The model under review builds one solid part; all positions refer to its coordinate system, in mm. A direction names the side the tool comes from. Round coordinates to 2 decimals unless told otherwise and drop trailing zeros. Write each loop counter-clockwise with the first axis right and the second up, starting at its lowest first coordinate (ties: lowest second). Pieces come first, ordered by that corner, then holes. Notation, with made-up numbers: (66, -40) - (70, -40) arc R30 cw to (70, -7) - close; hole circle Ø7 at (-5, -20.75). An arc over 180 degrees is marked (long way). One line per question, with ' | ' between items. Start each with the question number.
```python
from build123d import *

# Parameters (mm, degrees)
TABAN_FLAN_1_DEPTH = 10


# Sheet-metal steps are written as plain solids
with BuildPart() as part:
    # Çizim1 → Taban-Flanş1 (new body)
    with BuildSketch(Plane.XY):
        with BuildLine():
            Line((400, -35), (-400, -35))
            Line((-400, -35), (-400, 5))
            ThreePointArc((-400, 5), (-391.213203436, 26.213203436), (-370, 35))
            Line((-370, 35), (370, 35))
            ThreePointArc((370, 35), (391.213203436, 26.213203436), (400, 5))
            Line((400, 5), (400, -35))
        make_face()
        with BuildLine():
            Line((351, 20), (89, 20))
            ThreePointArc((89, 20), (75.564971157, 14.435028843), (70, 1))
            Line((70, 1), (70, -1))
            ThreePointArc((70, -1), (75.564971157, -14.435028843), (89, -20))
            Line((89, -20), (351, -20))
            ThreePointArc((351, -20), (364.435028843, -14.435028843), (370, -1))
            Line((370, -1), (370, 1))
            ThreePointArc((370, 1), (364.435028843, 14.435028843), (351, 20))
        make_face(mode=Mode.SUBTRACT)
        with BuildLine():
            Line((-70, 1), (-70, -1))
            ThreePointArc((-70, -1), (-75.564971157, -14.435028843), (-89, -20))
            Line((-89, -20), (-351, -20))
            ThreePointArc((-351, -20), (-364.435028843, -14.435028843), (-370, -1))
            Line((-370, -1), (-370, 1))
            ThreePointArc((-370, 1), (-364.435028843, 14.435028843), (-351, 20))
            Line((-351, 20), (-89, 20))
            ThreePointArc((-89, 20), (-75.564971157, 14.435028843), (-70, 1))
        make_face(mode=Mode.SUBTRACT)
    extrude(amount=-TABAN_FLAN_1_DEPTH)


solid = part.part
```
1. Add section B-B, the plane z = -2.75. Write out the cut boundary in (x, y).
2. Wall thickness on line 1 along X through (y, z) = (-0.5, -3.5); line 2 along Y through (x, z) = (-304, -7); line 3 along X through (y, z) = (11.5, -7.75): over which ranges is each line inside the solid? List them lowest first. Write a range as [from, to].
3. The part is to be moulded in two halves that separate along X. For faces 3 (the face through (6, 0, 0)), 4 (the face through (-364.29, -14.58, -4.93)), 5 (the face through (-391.445, 25.979, -4.93)), say which applies: pulls with the +X half, pulls with the -X half, needs draft (parallel to the pull), parting line crosses it, or undercut.
4. Machinability: for faces 1 (the face through (6, 0, -10)), 2 (the face through (-364.58, 14.29, -4.93)), which of the approach directions +Z, -Z, +X, -X, +Y, -Y give a long, thin tool a straight path to every point of the face, cutting with its end or side? Answer none if there is none.
5. Add section A-A, the plane x = -324. Write out the cut boundary in (y, z), then the cut area to 3 significant figures.
6. Add section C-C, the plane y = -9. Write out the cut boundary in (x, z), then the cut area to 3 significant figures.
Geometry check:
1) outline: (-400, -35) - (400, -35) - (400, 5) arc R30 ccw to (370, 35) - (-370, 35) arc R30 ccw to (-400, 5) - close; hole (-370, -1) arc R19 ccw to (-351, -20) - (-89, -20) arc R19 ccw to (-70, -1) - (-70, 1) arc R19 ccw to (-89, 20) - (-351, 20) arc R19 ccw to (-370, 1) - close; hole (70, -1) arc R19 ccw to (89, -20) - (351, -20) arc R19 ccw to (370, -1) - (370, 1) arc R19 ccw to (351, 20) - (89, 20) arc R19 ccw to (70, 1) - close
2) line 1: x = [-400, -370], [-70, 70], [370, 400] | line 2: y = [-35, -20], [20, 35] | line 3: x = [-399.29, -366.84], [-73.16, 73.16], [366.84, 399.29]
3) face 3: needs draft | face 4: undercut | face 5: pulls with the -X half
4) face 1: -Z, +X, -X, +Y, -Y | face 2: +Z, -Z
5) outline: (-35, -10) - (-20, -10) - (-20, 0) - (-35, 0) - close; (20, -10) - (35, -10) - (35, 0) - (20, 0) - close | area: 300 mm2
6) outline: (-400, -10) - (-368.23, -10) - (-368.23, 0) - (-400, 0) - close; (-71.77, -10) - (71.77, -10) - (71.77, 0) - (-71.77, 0) - close; (368.23, -10) - (400, -10) - (400, 0) - (368.23, 0) - close | area: 2,070 mm2
